```python
from build123d import *

# Parameters (mm, degrees)
SKETCH_1_R      = 2.5527
SKETCH_1_R_2    = 3.1
EXTRUDE_1_DEPTH = 3


with BuildPart() as part:
    # 草图1 → 凸台-拉伸1 (new body)
    with BuildSketch(Plane.XY):
        with BuildLine():
            Line((-431.8, 71.28685299), (-431.8, 146.05))
            ThreePointArc((-431.8, 146.05), (-426.7842688, 163.177211441), (-413.321803354, 174.893053509))
            ThreePointArc((-413.321803354, 174.893053509), (-409.712819047, 177.401355972), (-407.190786251, 181.000758638))
            ThreePointArc((-407.190786251, 181.000758638), (-406.894729782, 184.399778985), (-408.847840186, 187.197340155))
            ThreePointArc((-408.847840186, 187.197340155), (-409.896638803, 188.190326933), (-410.617854885, 189.441665672))
            ThreePointArc((-410.617854885, 189.441665672), (-418.564439883, 194.83685299), (-426.511139528, 189.44183454))
            ThreePointArc((-426.511139528, 189.44183454), (-428.349818055, 187.150121657), (-431.158279177, 186.28685299))
            Line((-431.158279177, 186.28685299), (-446.825059534, 186.28685299))
            ThreePointArc((-446.825059534, 186.28685299), (-449.633520657, 187.150121657), (-451.472199184, 189.44183454))
            ThreePointArc((-451.472199184, 189.44183454), (-459.722204594, 194.831468283), (-467.569172219, 188.870273751))
            ThreePointArc((-467.569172219, 188.870273751), (-468.928502541, 186.721457004), (-471.168900107, 185.519038159))
            Line((-471.168900107, 185.519038159), (-487.317425816, 181.644437971))
            ThreePointArc((-487.317425816, 181.644437971), (-490.249790032, 181.828630192), (-492.572411279, 183.628107117))
            ThreePointArc((-492.572411279, 183.628107117), (-500.567975463, 187.196951214), (-507.510215673, 181.861129284))
            ThreePointArc((-507.510215673, 181.861129284), (-509.113143283, 179.739691752), (-511.576958731, 178.739948001))
            ThreePointArc((-511.576958731, 178.739948001), (-515.326736937, 176.273665509), (-515.587539859, 171.793111105))
            ThreePointArc((-515.587539859, 171.793111105), (-510.367432741, 165.000898725), (-502.544116189, 161.511001094))
            ThreePointArc((-502.544116189, 161.511001094), (-484.948131906, 154.339092671), (-471.954869788, 140.474386658))
            ThreePointArc((-471.954869788, 140.474386658), (-468.883733752, 135.489867956), (-465.668015362, 130.59737795))
            Line((-465.668015362, 130.59737795), (-448.612101008, 69.509501917))
            ThreePointArc((-448.612101008, 69.509501917), (-439.40637216, 62.833958262), (-431.8, 71.28685299))
        make_face()
        with Locations((-459.418807983, 186.28685299)):
            Circle(SKETCH_1_R, mode=Mode.SUBTRACT)
        with Locations((-418.564530728, 186.28685299)):
            Circle(SKETCH_1_R, mode=Mode.SUBTRACT)
        with Locations((-499.563606874, 178.706147734)):
            Circle(SKETCH_1_R, mode=Mode.SUBTRACT)
        with Locations((-440.3, 71.28685299)):
            Circle(SKETCH_1_R_2, mode=Mode.SUBTRACT)
        with BuildLine():
            Line((-441.1092355, 106.511213318), (-441.1092355, 115.413429376))
            ThreePointArc((-441.1092355, 115.413429376), (-442.6967355, 118.163060033), (-445.8717355, 118.163060033))
            Line((-445.8717355, 118.163060033), (-453.581280756, 113.711952004))
            ThreePointArc((-453.581280756, 113.711952004), (-455.168780756, 110.962321347), (-453.581280756, 108.21269069))
            Line((-453.581280756, 108.21269069), (-445.8717355, 103.761582661))
            ThreePointArc((-445.8717355, 103.761582661), (-442.6967355, 103.761582661), (-441.1092355, 106.511213318))
        make_face(mode=Mode.SUBTRACT)
        with BuildLine():
            Line((-455.168781337, 116.461582661), (-447.459236081, 120.91269069))
            ThreePointArc((-447.459236081, 120.91269069), (-445.871736081, 123.662321347), (-447.459236081, 126.411952004))
            Line((-447.459236081, 126.411952004), (-455.168781337, 130.863060033))
            ThreePointArc((-455.168781337, 130.863060033), (-458.343781337, 130.863060033), (-459.931281337, 128.113429376))
            Line((-459.931281337, 128.113429376), (-459.931281337, 119.211213318))
            ThreePointArc((-459.931281337, 119.211213318), (-458.343781337, 116.461582661), (-455.168781337, 116.461582661))
        make_face(mode=Mode.SUBTRACT)
        with BuildLine():
            Line((-441.1092355, 157.311213318), (-441.1092355, 166.213429376))
            ThreePointArc((-441.1092355, 166.213429376), (-442.6967355, 168.963060033), (-445.8717355, 168.963060033))
            Line((-445.8717355, 168.963060033), (-453.581280756, 164.511952004))
            ThreePointArc((-453.581280756, 164.511952004), (-455.168780756, 161.762321347), (-453.581280756, 159.01269069))
            Line((-453.581280756, 159.01269069), (-445.8717355, 154.561582661))
            ThreePointArc((-445.8717355, 154.561582661), (-442.6967355, 154.561582661), (-441.1092355, 157.311213318))
        make_face(mode=Mode.SUBTRACT)
        with BuildLine():
            Line((-441.1092355, 131.911213318), (-441.1092355, 140.813429376))
            ThreePointArc((-441.1092355, 140.813429376), (-442.6967355, 143.563060033), (-445.8717355, 143.563060033))
            Line((-445.8717355, 143.563060033), (-453.581280756, 139.111952004))
            ThreePointArc((-453.581280756, 139.111952004), (-455.168780756, 136.362321347), (-453.581280756, 133.61269069))
            Line((-453.581280756, 133.61269069), (-445.8717355, 129.161582661))
            ThreePointArc((-445.8717355, 129.161582661), (-442.6967355, 129.161582661), (-441.1092355, 131.911213318))
        make_face(mode=Mode.SUBTRACT)
        with BuildLine():
            Line((-455.168781337, 141.861582661), (-447.459236081, 146.31269069))
            ThreePointArc((-447.459236081, 146.31269069), (-445.871736081, 149.062321347), (-447.459236081, 151.811952004))
            Line((-447.459236081, 151.811952004), (-455.168781337, 156.263060033))
            ThreePointArc((-455.168781337, 156.263060033), (-458.343781337, 156.263060033), (-459.931281337, 153.513429376))
            Line((-459.931281337, 153.513429376), (-459.931281337, 144.611213318))
            ThreePointArc((-459.931281337, 144.611213318), (-458.343781337, 141.861582661), (-455.168781337, 141.861582661))
        make_face(mode=Mode.SUBTRACT)
    extrude(amount=EXTRUDE_1_DEPTH)


solid = part.part
```
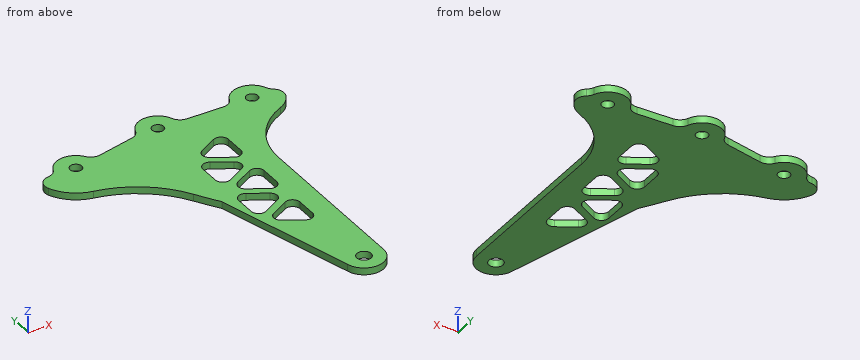
The listing builds one solid part. Answer for the finished solid, in the listing's coordinates (mm). Coordinates: 2 decimals unless noted, no trailing zeros. Write each loop counter-clockwise with the first axis right and the second up, starting at its lowest first coordinate (ties: lowest second). Pieces come first, ordered by that corner, then holes. Notation, with made-up numbers: M 89,-3.75 L 132,-3.75 A20 cw 132,1.25 Z; hole C 46,88 d1. An arc over 180 degrees is marked long. Use a Markdown table: item, result. Add a question column.
1. Given P1, Ø1.5, axis at y = 123.5, z = 1, coming from the +X side; P2, Ø1.5, axis at x = -439.5, z = 1.5, coming from the +Y side; P3, Ø3, axis at x = -499.56, y = 178.71, coming from the -Z side; P4, Ø1.5, axis at y = 150.5, z = 2, coming from the +X side, each flat-ended and moving along its own axis, determine where each tip first touches the part or whether it passes through.
2. Section C-C (z = 2.2) is taken. Count the separate pieces of the cut face and the enclosed holes in it, plus the area to 3 significant figures.
3. Section B-B (x = -417.5) is taken. Give the vertices of the cut face in (y, z), plus the area to 3 significant figures.
4. Section D-D (x = -504) is taken. Give the vertices of the cut face in (y, z), plus the area to 3 significant figures.
5. Section A-A (y = 122.5) is taken. Give the vertices of the cut face in (x, z), plus the area to 3 significant figures.
6. Straight lines are drawn through the part: line 1 along X through (y, z) = (156, 1.5); line 2 along Y through (x, z) = (-440.3, 1.7); line 3 along X through (y, z) = (186, 0.3). For each, find the intervals that lie inside material, in ascending order. Write a range as [from, to].
Data:
| question | item | result |
|---|---|---|
| 1 | P1 | stops at x = -431.8 |
| 1 | P2 | stops at y = 186.29 |
| 1 | P3 | passes through |
| 1 | P4 | stops at x = -431.37 |
| 2 | separate pieces | 1 |
| 2 | enclosed holes | 9 |
| 2 | area | 4,770 mm2 |
| 3 | outline | M 172.57,0 L 183.97,0 L 183.97,3 L 172.57,3 Z; M 188.61,0 L 194.77,0 L 194.77,3 L 188.61,3 Z |
| 3 | area | 52.7 mm2 |
| 4 | outline | M 161.83,0 L 186.02,0 L 186.02,3 L 161.83,3 Z |
| 4 | area | 72.6 mm2 |
| 5 | outline | M -463.41,0 L -459.93,0 L -459.93,3 L -463.41,3 Z; M -446.09,0 L -431.8,0 L -431.8,3 L -446.09,3 Z |
| 5 | area | 53.3 mm2 |
| 6 | line 1 | x = [-487.55, -458.73], [-454.71, -448.36], [-441.39, -430.2] |
| 6 | line 2 | y = [62.79, 68.19], [74.39, 186.29] |
| 6 | line 3 | x = [-504.02, -495.1], [-469.93, -461.96], [-456.88, -421.1], [-416.03, -407.65] |
